```python
from build123d import *

# Parameters (mm, degrees)
BOSS_EXTRUDE3_DEPTH     = 10
SKETCH3_W               = 43.8640004
SKETCH3_H               = 10
BOSS_EXTRUDE4_DEPTH     = 21
SKETCH4_R               = 2
CUT_EXTRUDE1_DEPTH      = 83.054859698
SKETCH5_R               = 3.5
CUT_EXTRUDE2_DEPTH      = 4
FILLET1_R               = 2
FILLET2_R               = 2
FILLET3_R               = 2
FILLET4_R               = 2
CUT_EXTRUDE3_DEPTH      = 69.769542741
CUT_EXTRUDE3_DEPTH_BACK = 69.769542741
SKETCH6_R               = 2.5
FILLET5_R               = 10
FILLET6_R               = 10
SKETCH7_R               = 4.5
CUT_EXTRUDE4_DEPTH      = 10
CUT_EXTRUDE5_START      = 10
SKETCH8_R               = 4.5
CUT_EXTRUDE5_DEPTH      = 10


# Some blends are built 0.0001 mm under size
with BuildPart() as part:
    # Sketch2 → Boss-Extrude3 (new body)
    with BuildSketch(Plane.XY):
        with BuildLine():
            Line((-44, -2.5), (-44, -6.5))
            Line((-44, -6.5), (-33.372893192, -6.5))
            ThreePointArc((-33.372893192, -6.5), (22.19279887, -25.758099276), (11.3640004, 32.04464846))
            Line((11.3640004, 32.04464846), (11.3640004, 42))
            Line((11.3640004, 42), (-32.5, 42))
            Line((-32.5, 42), (-32.5, 9.987492178))
            ThreePointArc((-32.5, 9.987492178), (-32.982573653, 8.255291346), (-33.372893192, 6.5))
            Line((-33.372893192, 6.5), (-44, 6.5))
            Line((-44, 6.5), (-44, 2.5))
            Line((-44, 2.5), (-28.892040426, 2.5))
            ThreePointArc((-28.892040426, 2.5), (29, 0), (-28.892040426, -2.5))
            Line((-28.892040426, -2.5), (-44, -2.5))
        make_face()
    extrude(amount=BOSS_EXTRUDE3_DEPTH)

    # Sketch3 → Boss-Extrude4 (add)
    with BuildSketch(Plane(origin=(0, 0, 0), x_dir=(-1, 0, 0), z_dir=(0, 0, -1))):
        with Locations((10.5679998, 37)):
            Rectangle(SKETCH3_W, SKETCH3_H)
    extrude(amount=-BOSS_EXTRUDE4_DEPTH)

    # Sketch4 → Cut-Extrude1 (cut, through all)
    with BuildSketch(Plane.XZ.offset(-32)):
        with Locations(Location((-26.5, 15.5, 0), (0, 0, 270))):
            Circle(SKETCH4_R)
        with Locations(Location((-10.5, 15.5, 0), (0, 0, 270))):
            Circle(SKETCH4_R)
    extrude(amount=-CUT_EXTRUDE1_DEPTH, mode=Mode.SUBTRACT)

    # Sketch5 → Cut-Extrude2 (cut)
    with BuildSketch(Plane.XZ.offset(-32)):
        with Locations(Location((-26.5, 15.5, 0), (0, 0, 270))):
            Circle(SKETCH5_R)
        with Locations(Location((-10.5, 15.5, 0), (0, 0, 270))):
            Circle(SKETCH5_R)
    extrude(amount=-CUT_EXTRUDE2_DEPTH, mode=Mode.SUBTRACT)

    # Fillet1
    fillet1_edges = [part.edges().sort_by_distance(p)[0] for p in [
        (-10.5679998, 32, 10),
    ]]
    fillet(fillet1_edges, radius=FILLET1_R - 0.0001)  # a hair under: the kernel refuses the full size

    # Fillet2
    # the kernel refuses this fillet: 2 mm, written as the material it takes off along each edge
    with BuildSketch(Plane(origin=(11.3640004, 30.0001, 11.9999), x_dir=(0, -0.597567009658115, 0.8018189751859569), z_dir=(0, 0.8018189751859569, 0.597567009658115))) as fillet2_piece_1_section:
        with BuildLine():
            CenterArc((1.9999 + FILLET2_R, -FILLET2_R), FILLET2_R, 90, 90)
            Line((1.9999 + FILLET2_R, 0), (1.9999, 0))
            Line((1.9999, 0), (1.9999, -FILLET2_R))
        make_face()
    fillet2_piece_1 = revolve(axis=Axis((11.3640004, 30.0001, 11.9999), (1, 0, 0)), revolution_arc=233.304154445, mode=Mode.PRIVATE)
    fillet2_piece_1 = split(fillet2_piece_1, bisect_by=Plane(origin=(10.740737353, 31.499904871, 10), z_dir=(0, 0, 1)), keep=Keep.TOP, mode=Mode.PRIVATE)
    add(fillet2_piece_1, mode=Mode.SUBTRACT)
    with BuildSketch(Plane(origin=(11.3640004, 30.0001, 11.9999), x_dir=(0, -0.597567009658115, 0.8018189751859569), z_dir=(0, 0.8018189751859569, 0.597567009658115))) as fillet2_piece_2_section:
        with BuildLine():
            CenterArc((1.9999 + FILLET2_R, -FILLET2_R), FILLET2_R, 90, 90)
            Line((1.9999 + FILLET2_R, 0), (1.9999, 0))
            Line((1.9999, 0), (1.9999, -FILLET2_R))
        make_face()
    fillet2_piece_2 = revolve(axis=Axis((11.3640004, 30.0001, 11.9999), (1, 0, 0)), revolution_arc=233.304154445, mode=Mode.PRIVATE)
    fillet2_piece_2 = fillet2_piece_2 - Plane(origin=(0, 0, 9.683888081), x_dir=(-0.9815556821156025, -0.19117647058823523, 0), z_dir=(0, 0, -1)) * Cylinder(34, 16, mode=Mode.PRIVATE)
    add(fillet2_piece_2, mode=Mode.SUBTRACT)
    with BuildSketch(Plane(origin=(11.3640004, 32, 11.9999), x_dir=(-1, 0, 0), z_dir=(0, 0, 1))) as fillet2_piece_3:
        with BuildLine():
            CenterArc((FILLET2_R, -FILLET2_R), FILLET2_R, 90, 90)
            Line((0, -FILLET2_R), (0, 0))
            Line((0, 0), (FILLET2_R, 0))
        make_face()
    extrude(amount=14.0001, mode=Mode.SUBTRACT)

    # Fillet3
    fillet3_edges = [part.edges().sort_by_distance(p)[0] for p in [
        (-32.5, 31.414242852, 10.585757148),
        (-32.5, 19.993796089, 10),
        (-32.5, 32, 16.49995),
    ]]
    fillet(fillet3_edges, radius=FILLET3_R)

    # Fillet4
    fillet4_edges = [part.edges().sort_by_distance(p)[0] for p in [
        (-10.5679998, 32, 21),
        (10.778213962, 32.585786438, 21),
        (-32.5, 38, 21),
        (-31.914213562, 32.585786438, 21),
        (11.3640004, 38, 21),
    ]]
    fillet(fillet4_edges, radius=FILLET4_R - 0.0001)  # a hair under: the kernel refuses the full size

    # Sketch6 → Cut-Extrude3 (cut, two sides: drawn at the far end of the back side and taken through both)
    with BuildSketch(Plane.XZ.offset(6.5).offset(-CUT_EXTRUDE3_DEPTH_BACK)):
        with Locations(Location((-38.686446596, 5, 0), (0, 0, 270))):
            Circle(SKETCH6_R)
    extrude(amount=CUT_EXTRUDE3_DEPTH + CUT_EXTRUDE3_DEPTH_BACK, mode=Mode.SUBTRACT)

    # Fillet5
    # the kernel refuses this fillet: 10 mm, written as the material it adds along each edge
    with BuildSketch(Plane(origin=(-33.372893192, -6.5, 0), x_dir=(0.28439822949725985, -0.9587062360592132, 0), z_dir=(0, 0, 1))) as fillet5_piece_1_section:
        with BuildLine():
            CenterArc((7.477908641, -9.953938032), FILLET5_R, 95.501431601, 67.975687163)
            Line((-2.109153719, -7.109955737), (0, 0))
            ThreePointArc((0, 0), (3.259601203, -0.15661069), (6.519202405, 0))
        make_face()
    fillet5_piece_1 = extrude(amount=10, mode=Mode.PRIVATE)
    fillet5_piece_1 = fillet5_piece_1 - Plane(origin=(-38.686446596, -7.980864668, 5), x_dir=(0, 0, -1), z_dir=(0, -1, 0)) * Cylinder(2.5, 49, mode=Mode.PRIVATE)
    add(fillet5_piece_1)

    # Fillet6
    # the kernel refuses this fillet: 10 mm, written as the material it adds along each edge
    with BuildSketch(Plane(origin=(-33.372893192, 6.5, 0), x_dir=(0.28439822949726035, 0.9587062360592132, 0), z_dir=(0, 0, 1))) as fillet6_piece_1_section:
        with BuildLine():
            CenterArc((7.477908641, 9.953938032), FILLET6_R, 196.522881236, 67.975687163)
            Line((-2.109153719, 7.109955737), (0, 0))
            ThreePointArc((0, 0), (3.259601203, 0.15661069), (6.519202405, 0))
        make_face()
    fillet6_piece_1 = extrude(amount=10, mode=Mode.PRIVATE)
    fillet6_piece_1 = fillet6_piece_1 - Plane(origin=(-38.686446596, 7.980864668, 5), x_dir=(0, 0, -1), z_dir=(0, -1, 0)) * Cylinder(2.5, 49, mode=Mode.PRIVATE)
    add(fillet6_piece_1)

    # Sketch7 → Cut-Extrude4 (cut)
    with BuildSketch(Plane.XZ.offset(6.5)):
        with Locations((-38.686446596, 5)):
            Circle(SKETCH7_R)
    extrude(amount=CUT_EXTRUDE4_DEPTH, mode=Mode.SUBTRACT)

    # Sketch8 → Cut-Extrude5 (cut)
    with BuildSketch(Plane(origin=(0, 6.5, 0), x_dir=(1, 0, 0), z_dir=(0, 1, 0)).offset(CUT_EXTRUDE5_START)):
        with Locations((-38.686446596, -5)):
            Circle(SKETCH8_R)
    extrude(amount=-CUT_EXTRUDE5_DEPTH, mode=Mode.SUBTRACT)


solid = part.part
```
Input: part model. Units: mm. Frame: model coordinates. A direction names the side the tool comes from. Round coordinates to 2 decimals unless told otherwise and drop trailing zeros. Loops run counter-clockwise (first coordinate to the right, second up) from the corner with the lowest first, then second, coordinate; pieces in that order, holes last.
1) Material intervals for line 1 (X direction, y = 40.55, z = 15.5); line 2 (Y direction, x = 0, z = 6.75); line 3 (X direction, y = -4, z = 6.5), sorted ascending.
Ans:
line 1: x = -32.5 to -28.5, -24.5 to -12.5, -8.5 to 11.36
line 2: y = -34 to -29, 29 to 42
line 3: x = -44 to -40.69, -36.69 to -28.72, 28.72 to 33.76
2) Pull-direction query (Z, two-part tool) for faces 1 (the cylindrical face through (-34.19, -7.45, 4.87)), 2 (the cylindrical face through (-10.29, 31.43, 10.6)), 3 (the flat face through (-44, 5, 5)); classes: released by +Z, released by -Z, zero draft, split by the parting line, or undercut.
Ans:
face 1: undercut
face 2: released by +Z
face 3: zero draft
3) Section query C-C on y = -11. Return the cut outline in (x, z), plus the area to 3 significant figures.
Ans:
outline: (-32.44, 0) - (-26.83, 0) - (-26.83, 10) - (-32.44, 10) - close; (26.83, 0) - (32.17, 0) - (32.17, 10) - (26.83, 10) - close
area: 109 mm2
4) Set-up query: faces 4 (the cylindrical face through (-31.93, 32.6, 15.45)), 5 (the flat face through (-26, 36, 13)), 6 (the flat face through (-32.5, 30, 7)). Return all of +Z, -Z, +X, -X, +Y, -Y with unobstructed straight access to the full face (end or side cutting, diameter ignored); none if empty.
Ans:
face 4: +Z, -X, -Y
face 5: -Y
face 6: +Z, -Z, -X, +Y
5) Pin query (flat end, axial travel): pin 1 (9.5 mm diameter, centred on y = 19, z = 10.5, fed in from -X); pin 2 (11.5 mm diameter, centred on x = -38.69, z = 5, fed in from -Y); pin 3 (6.5 mm diameter, centred on x = -38.69, z = 5, fed in from +Y); pin 4 (11 mm diameter, centred on x = -10.5, z = 15.5, fed in from +Y). Return the tip coordinate at first contact, or that it passes through.
Ans:
pin 1: stops at x = -32.5
pin 2: stops at y = -10.3
pin 3: stops at y = 6.5
pin 4: stops at y = 42
6) Section query D-D on z = 5. Return the cut outline in (x, y), plus the area to 3 significant figures.
Ans:
outline: (-44, -6.5) - (-41.19, -6.5) - (-41.19, -2.5) - (-44, -2.5) - close; (-44, 2.5) - (-41.19, 2.5) - (-41.19, 6.5) - (-44, 6.5) - close; (-36.19, -6.5) - (-34.19, -6.5) - (-34.19, -8.99) arc R10 cw to (-31.52, -12.75) arc R34 ccw (long way) to (11.36, 32.04) - (11.36, 42) - (-32.5, 42) - (-32.5, 10.91) arc R10 cw to (-34.19, 8.99) - (-34.19, 6.5) - (-36.19, 6.5) - (-36.19, 2.5) - (-28.89, 2.5) arc R29 cw (long way) to (-28.89, -2.5) - (-36.19, -2.5) - close
area: 1,580 mm2
7) Section query A-A on z = 15.5. Return the cut outline in (x, y).
Ans:
outline: (-32.5, 34) arc R2 ccw to (-30.5, 32) - (-30, 32) - (-30, 36) - (-28.5, 36) - (-28.5, 42) - (-32.5, 42) - close; (-24.5, 36) - (-23, 36) - (-23, 32) - (-14, 32) - (-14, 36) - (-12.5, 36) - (-12.5, 42) - (-24.5, 42) - close; (-8.5, 36) - (-7, 36) - (-7, 32) - (9.36, 32) arc R2 ccw to (11.36, 34) - (11.36, 42) - (-8.5, 42) - close
8) Section query B-B on x = 0. Return the cut outline in (y, z), plus the area to 3 significant figures.
Ans:
outline: (-34, 0) - (-29, 0) - (-29, 10) - (-34, 10) - close; (29, 0) - (42, 0) - (42, 21) - (34, 21) arc R2 ccw to (32, 19) - (32, 12) arc R2 cw to (30, 10) - (29, 10) - close
area: 290 mm2
